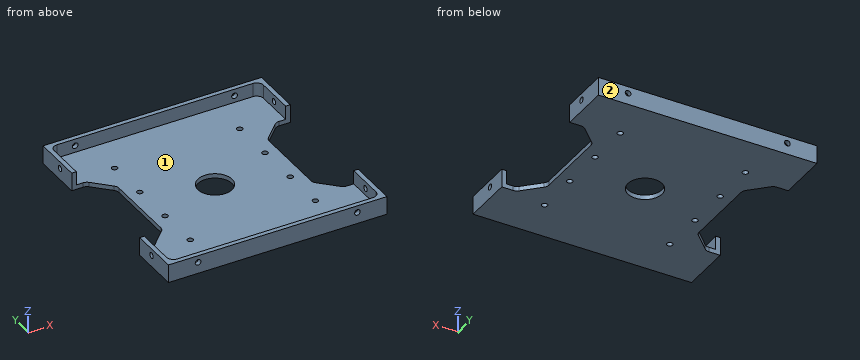
from build123d import *

# Parameters (mm, degrees)
SKETCH1_W                      = 96
SKETCH1_H                      = 96
BOSS_EXTRUDE1_DEPTH            = 8
SKETCH2_W                      = 92
SKETCH2_H                      = 92
COMPONENT_PLATFORM_DEPTH       = 6
CABLE_SLOTS_DEPTH              = 6
SKETCH4_R                      = 7.5
CENTER_MASS_CUT_DEPTH          = 6
INNER_CORNER_FILLETS_R         = 3
M3X0_5_TAPPED_HOLE1_AT_2_COUNT = 2
M3X0_5_TAPPED_HOLE1_AT_2_PITCH = 70
M3X0_5_TAPPED_HOLE2_AT_2_COUNT = 2
M3X0_5_TAPPED_HOLE2_AT_2_PITCH = 70
M3X0_5_TAPPED_HOLE3_D          = 2.5


with BuildPart() as part:
    # Sketch1 → Boss-Extrude1 (new body)
    with BuildSketch(Plane.XY):
        Rectangle(SKETCH1_W, SKETCH1_H)
    extrude(amount=BOSS_EXTRUDE1_DEPTH)

    # Sketch2 → Component Platform (cut)
    with BuildSketch(Plane.XY.offset(8)):
        Rectangle(SKETCH2_W, SKETCH2_H)
    extrude(amount=-COMPONENT_PLATFORM_DEPTH, mode=Mode.SUBTRACT)

    # Sketch3 → Cable Slots (cut, symmetric)
    with BuildSketch(Plane.XY.offset(2)):
        with BuildLine():
            Line((-40.878679656, -25.121320344), (-33.878679656, -18.121320344))
            ThreePointArc((-33.878679656, -18.121320344), (-33.228361402, -17.148050297), (-33, -16))
            Line((-33, -16), (-33, 16))
            ThreePointArc((-33, 16), (-33.228361402, 17.148050297), (-33.878679656, 18.121320344))
            Line((-33.878679656, 18.121320344), (-40.878679656, 25.121320344))
            ThreePointArc((-40.878679656, 25.121320344), (-41.851949703, 25.771638598), (-43, 26))
            Line((-43, 26), (-48, 26))
            Line((-48, 26), (-48, -26))
            Line((-48, -26), (-43, -26))
            ThreePointArc((-43, -26), (-41.851949703, -25.771638598), (-40.878679656, -25.121320344))
        make_face()
        with BuildLine():
            Line((48, -26), (48, 26))
            Line((48, 26), (43, 26))
            ThreePointArc((43, 26), (41.851949703, 25.771638598), (40.878679656, 25.121320344))
            Line((40.878679656, 25.121320344), (33.878679656, 18.121320344))
            ThreePointArc((33.878679656, 18.121320344), (33.228361402, 17.148050297), (33, 16))
            Line((33, 16), (33, -16))
            ThreePointArc((33, -16), (33.228361402, -17.148050297), (33.878679656, -18.121320344))
            Line((33.878679656, -18.121320344), (40.878679656, -25.121320344))
            ThreePointArc((40.878679656, -25.121320344), (41.851949703, -25.771638598), (43, -26))
            Line((43, -26), (48, -26))
        make_face()
    extrude(amount=CABLE_SLOTS_DEPTH, both=True, mode=Mode.SUBTRACT)

    # Sketch4 → Center Mass Cut (cut)
    with BuildSketch(Plane.XY.offset(2)):
        Circle(SKETCH4_R)
    extrude(amount=-CENTER_MASS_CUT_DEPTH, mode=Mode.SUBTRACT)

    # Inner Corner Fillets
    inner_corner_fillets_edges = [part.edges().sort_by_distance(p)[0] for p in [
        (-46, -46, 5),
        (-46, 46, 5),
        (46, 46, 5),
        (46, -46, 5),
    ]]
    fillet(inner_corner_fillets_edges, radius=INNER_CORNER_FILLETS_R)

    # Sketch10 → M3x0.5 Tapped Hole1 (revolve, cut)
    with BuildSketch(Plane(origin=(48, -35, 5), x_dir=(0, 0, -1), z_dir=(0, 1, 0))):
        Polygon((0, 0), (0, 10.751075774), (1.25, 10), (1.25, 0), align=None)
    m3x0_5_tapped_hole1 = revolve(axis=Axis((54.35, -35, 5), (-1, 0, 0)), mode=Mode.SUBTRACT)

    # M3x0.5 Tapped Hole1 at 2: M3x0.5 Tapped Hole1 ×2
    with Locations(*[(0, i * M3X0_5_TAPPED_HOLE1_AT_2_PITCH, 0) for i in range(1, M3X0_5_TAPPED_HOLE1_AT_2_COUNT)]):
        add(m3x0_5_tapped_hole1, mode=Mode.SUBTRACT)

    # Sketch13 → M3x0.5 Tapped Hole2 (revolve, cut)
    with BuildSketch(Plane(origin=(-35, -48, 5), x_dir=(0, 0, -1), z_dir=(1, 0, 0))):
        Polygon((0, 0), (0, 10.751075774), (1.25, 10), (1.25, 0), align=None)
    m3x0_5_tapped_hole2 = revolve(axis=Axis((-35, -54.35, 5), (0, 1, 0)), mode=Mode.SUBTRACT)

    # M3x0.5 Tapped Hole2 at 2: M3x0.5 Tapped Hole2 ×2
    with Locations(*[(i * M3X0_5_TAPPED_HOLE2_AT_2_PITCH, 0, 0) for i in range(1, M3X0_5_TAPPED_HOLE2_AT_2_COUNT)]):
        add(m3x0_5_tapped_hole2, mode=Mode.SUBTRACT)

    # Mirror1: M3x0.5 Tapped Hole1 across plane
    add(m3x0_5_tapped_hole1.mirror(Plane(origin=(0, 0, 0), x_dir=(0, 0, 1), z_dir=(1, 0, 0))), mode=Mode.SUBTRACT)

    # Mirror1 copy 1 sketch → Mirror1 copy 1 (revolve, cut)
    with BuildSketch(Plane(origin=(-48, 35, 5), x_dir=(0, 0, -1), z_dir=(0, 1, 0))):
        Polygon((0, 0), (0, -10.751075774), (1.25, -10), (1.25, 0), align=None)
    revolve(axis=Axis((-54.35, 35, 5), (-1, 0, 0)), mode=Mode.SUBTRACT)

    # Mirror2: M3x0.5 Tapped Hole2 across plane
    add(m3x0_5_tapped_hole2.mirror(Plane(origin=(0, 0, 0), x_dir=(0, 0, 1), z_dir=(0, -1, 0))), mode=Mode.SUBTRACT)

    # Mirror2 copy 1 sketch → Mirror2 copy 1 (revolve, cut)
    with BuildSketch(Plane(origin=(35, 48, 5), x_dir=(0, 0, -1), z_dir=(1, 0, 0))):
        Polygon((0, 0), (0, -10.751075774), (1.25, -10), (1.25, 0), align=None)
    revolve(axis=Axis((35, 54.35, 5), (0, 1, 0)), mode=Mode.SUBTRACT)

    # M3x0.5 Tapped Hole3 (through all)
    with Locations(Plane.XY.offset(2)):
        with Locations((-27.5, 28.95), (-27.5, 9.65), (-27.5, -9.65), (-27.5, -28.95), (27.5, -28.95), (27.5, -9.65), (27.5, 9.65), (27.5, 28.95)):
            Hole(M3X0_5_TAPPED_HOLE3_D / 2)


solid = part.part
The model under review builds one solid part; all positions refer to its coordinate system, in mm. Face numbers are marked on the shaded views. Round coordinates to 2 decimals unless told otherwise and drop trailing zeros. Loops run counter-clockwise (first coordinate to the right, second up) from the corner with the lowest first, then second, coordinate; pieces in that order, holes last. Notation, with made-up numbers: (39.25, 82.25) -> (58.25, 82.25) arc R9 ccw to (58.25, 92.25) -> close; hole circle Ø4 at (57, 87). An arc over 180 degrees is marked (long way). Write item = value, one per line. Start each with the question number.
Item 1: To check wall thickness, follow L1, parallel to X at y = -47.55, z = 5; L2, parallel to Y at x = -27.5, z = 0.95; L3, parallel to X at y = 39, z = 2.5. State the ranges of each line that lie inside material, in increasing order.
Item 2: Mouldability with a two-part tool opening along X and no side actions: class the marked faces 1 and 2 as released by +X, released by -X, zero draft, split by the parting line, or undercut.
Item 3: Take a section at B-B on x = -6. Give the boundary of the cut face in (y, z), plus the area to 3 significant figures.
Item 4: Take a section at C-C on y = 0. Give the boundary of the cut face in (x, z), plus the area to 3 significant figures.
Item 5: Take a section at D-D on x = -27.5. Give the boundary of the cut face in (y, z).
Item 6: Insertion check: pin 1 (3 mm diameter, centred on x = -22, y = -18, fed in from +Z); pin 2 (1 mm diameter, centred on y = -7, z = 1.5, fed in from +X). Each pin has a flat end and moves straight along its axis. Give the tip position at first contact, or say it passes through.
Item 7: Take a section at A-A on y = -28.95. Give the boundary of the cut face in (x, z).
Result:
q1.L1 = -48 to -36.25, -33.75 to 33.75, 36.25 to 48
q1.L2 = -48 to -30.2, -27.7 to -10.9, -8.4 to 8.4, 10.9 to 27.7, 30.2 to 48
q1.L3 = -48 to -46, 46 to 48
q2.face_1 = undercut
q2.face_2 = zero draft
q3.outline = (-48, 0) -> (-4.5, 0) -> (-4.5, 2) -> (-46, 2) -> (-46, 8) -> (-48, 8) -> close; (4.5, 0) -> (48, 0) -> (48, 8) -> (46, 8) -> (46, 2) -> (4.5, 2) -> close
q3.area = 198 mm²
q4.outline = (-33, 0) -> (-7.5, 0) -> (-7.5, 2) -> (-33, 2) -> close; (7.5, 0) -> (33, 0) -> (33, 2) -> (7.5, 2) -> close
q4.area = 102 mm²
q5.outline = (-48, 0) -> (-30.2, 0) -> (-30.2, 2) -> (-46, 2) -> (-46, 8) -> (-48, 8) -> close; (-27.7, 0) -> (-10.9, 0) -> (-10.9, 2) -> (-27.7, 2) -> close; (-8.4, 0) -> (8.4, 0) -> (8.4, 2) -> (-8.4, 2) -> close; (10.9, 0) -> (27.7, 0) -> (27.7, 2) -> (10.9, 2) -> close; (30.2, 0) -> (48, 0) -> (48, 8) -> (46, 8) -> (46, 2) -> (30.2, 2) -> close
q6.pin_1 = 2
q6.pin_2 = 33
q7.outline = (-48, 0) -> (-28.75, 0) -> (-28.75, 2) -> (-46, 2) -> (-46, 8) -> (-48, 8) -> close; (-26.25, 0) -> (26.25, 0) -> (26.25, 2) -> (-26.25, 2) -> close; (28.75, 0) -> (48, 0) -> (48, 8) -> (46, 8) -> (46, 2) -> (28.75, 2) -> close
